Drawing for the job (mm, zero at the part's lowest x, y, z). A direction names the side the tool comes from. Round coordinates to 2 decimals unless told otherwise and drop trailing zeros. Write each loop counter-clockwise with the first axis right and the second up, starting at its lowest first coordinate (ties: lowest second). Pieces come first, ordered by that corner, then holes. Notation, with made-up numbers: (0, 48) -> (56, 48) arc R27 ccw to (56, 69) -> close; hole circle Ø1 at (67.25, 31.25). An arc over 180 degrees is marked (long way). One line per question, with ' | ' between items.
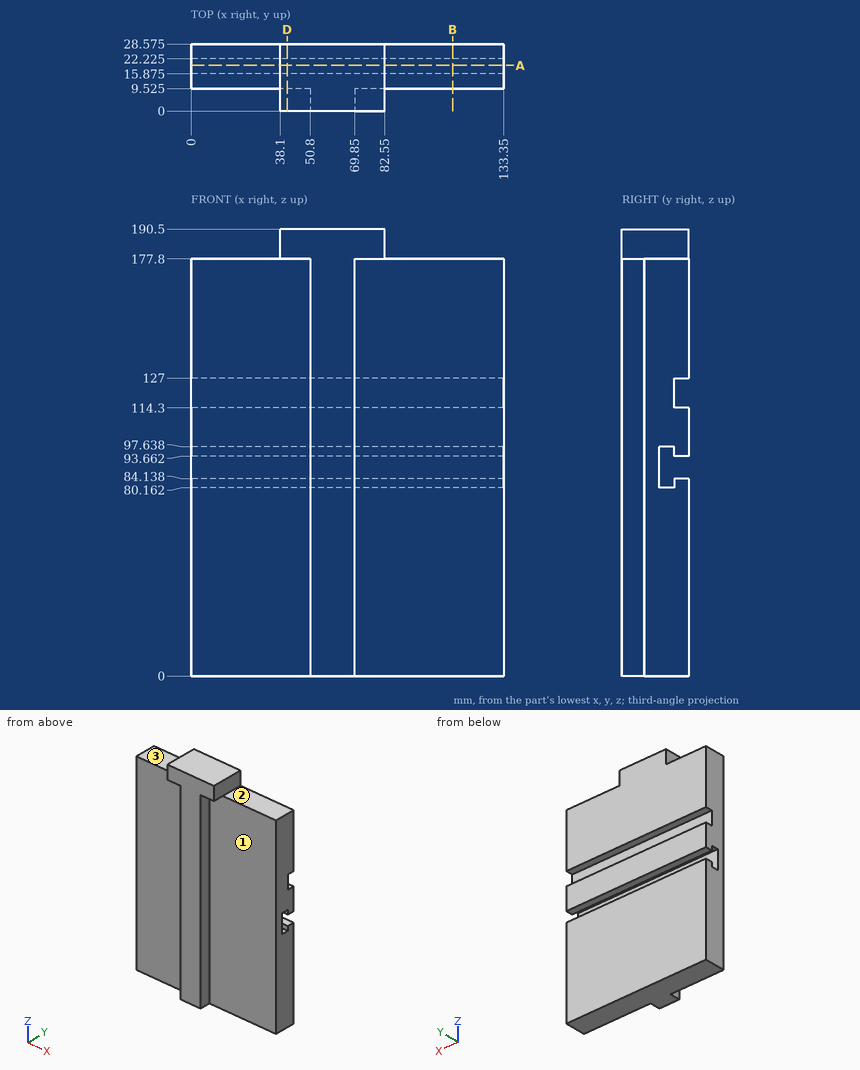
(1) 3-axis set-ups, long thin cutter, end or side, ignore diameter. For the marked faces 1, 2 and 3: which of +Z, -Z, +X, -X, +Y, -Y reach the whole face in a straight line?
Calculated:
face 1: -Z, +X, -Y | face 2: +Z, +X, +Y, -Y | face 3: +Z, -X, +Y, -Y
(2) Slice it at D-D (x = 41). Write the cut outline in (y, z) (1 decimal), then the cut area to 3 significant figures.
Calculated:
outline: (0, 177.8) -> (9.5, 177.8) -> (9.5, 0) -> (28.6, 0) -> (28.6, 84.1) -> (22.2, 84.1) -> (22.2, 80.2) -> (15.9, 80.2) -> (15.9, 97.6) -> (22.2, 97.6) -> (22.2, 93.7) -> (28.6, 93.7) -> (28.6, 114.3) -> (22.2, 114.3) -> (22.2, 127) -> (28.6, 127) -> (28.6, 190.5) -> (0, 190.5) -> close | area: 3,500 mm2
(3) Slice it at A-A (y = 19.5). Write the cut outline in (x, z).
Calculated:
outline: (0, 0) -> (133.35, 0) -> (133.35, 80.16) -> (0, 80.16) -> close; (0, 97.64) -> (133.35, 97.64) -> (133.35, 177.8) -> (82.55, 177.8) -> (82.55, 190.5) -> (38.1, 190.5) -> (38.1, 177.8) -> (0, 177.8) -> close
(4) Drop flat-ended pins along their axis: pin 1 (1.9 mm diameter, centred on x = 35.5, y = 19, fed in from +Z); pin 2 (3 mm diameter, centred on y = 6, z = 69.5, fed in from +X); pin 3 (7.5 mm diameter, centred on y = 3, z = 53, fed in from -X). Give the stop position or say it passes through.
Calculated:
pin 1: z = 177.8 | pin 2: x = 69.85 | pin 3: x = 50.8
(5) Slice it at B-B (x = 111.5). Write the cut outline in (y, z) (1 decimal).
Calculated:
outline: (9.5, 0) -> (28.6, 0) -> (28.6, 84.1) -> (22.2, 84.1) -> (22.2, 80.2) -> (15.9, 80.2) -> (15.9, 97.6) -> (22.2, 97.6) -> (22.2, 93.7) -> (28.6, 93.7) -> (28.6, 114.3) -> (22.2, 114.3) -> (22.2, 127) -> (28.6, 127) -> (28.6, 177.8) -> (9.5, 177.8) -> close
(6) Wall check: line 1 (Z direction, x = 67, y = 23.25); line 2 (Z direction, x = 115, y = 19.5); line 3 (Z direction, x = 104.5, y = 25.5). Give the ranges that are in metal, low to high. Write a range as from..to.
Calculated:
line 1: 0..84.14, 93.66..114.3, 127..190.5 | line 2: 0..80.16, 97.64..177.8 | line 3: 0..84.14, 93.66..114.3, 127..177.8
